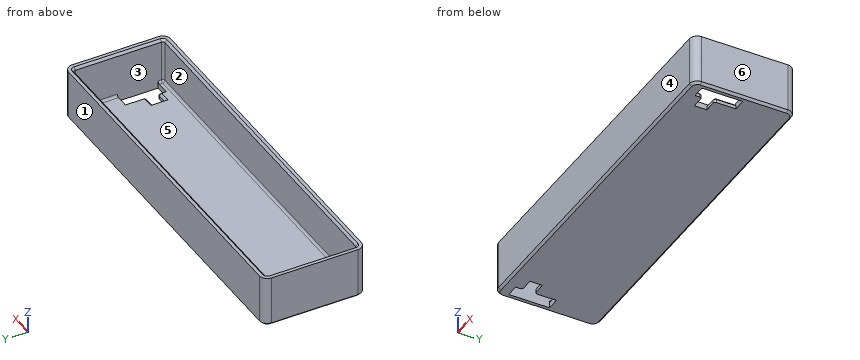
from build123d import *

# Parameters (mm, degrees)
SKETCH_W        = 154
SKETCH_H        = 40
PAD_DEPTH       = 2.5
SKETCH001_W     = 154
SKETCH001_H     = 22.5
PAD001_DEPTH    = 2.5
SKETCH002_W     = 154
SKETCH002_H     = 22.5
PAD002_DEPTH    = 2.5
SKETCH003_W     = 45
SKETCH003_H     = 22.5
PAD003_DEPTH    = 2.5
SKETCH004_W     = 45
SKETCH004_H     = 22.5
PAD004_DEPTH    = 2.5
SKETCH005_W     = 5.5
SKETCH005_H     = 18
POCKET_DEPTH    = 5
SKETCH006_W     = 6
SKETCH006_H     = 5.5
POCKET001_DEPTH = 5
FILLET_R        = 1
CHAMFER_SIZE    = 1
FILLET001_R     = 1
CHAMFER001_SIZE = 1
FILLET002_R     = 1
FILLET003_R     = 3.5
CHAMFER002_SIZE = 1
CHAMFER003_SIZE = 1


with BuildPart() as part:
    # Sketch → Pad (new body)
    with BuildSketch(Plane.XY):
        Rectangle(SKETCH_W, SKETCH_H)
    extrude(amount=PAD_DEPTH)

    # Sketch001 (on Face2 of Pad) → Pad001 (join)
    with BuildSketch(Plane.XZ.offset(20)):
        with Locations((0, 11.25)):
            Rectangle(SKETCH001_W, SKETCH001_H)
    extrude(amount=PAD001_DEPTH)

    # Sketch002 (on Face1 of Pad001) → Pad002 (join)
    with BuildSketch(Plane(origin=(0, 20, 0), x_dir=(-1, 0, 0), z_dir=(0, 1, 0))):
        with Locations((0, 11.25)):
            Rectangle(SKETCH002_W, SKETCH002_H)
    extrude(amount=PAD002_DEPTH)

    # Sketch003 (on Face9 of Pad002) → Pad003 (join)
    with BuildSketch(Plane.YZ.offset(77)):
        with Locations((0, 11.25)):
            Rectangle(SKETCH003_W, SKETCH003_H)
    extrude(amount=PAD003_DEPTH)

    # Sketch004 (on Face4 of Pad003) → Pad004 (join)
    with BuildSketch(Plane(origin=(-77, 0, 0), x_dir=(0, -1, 0), z_dir=(-1, 0, 0))):
        with Locations((0, 11.25)):
            Rectangle(SKETCH004_W, SKETCH004_H)
    extrude(amount=PAD004_DEPTH)

    # Sketch005 (on Face10 of Pad004) → Pocket (cut)
    with BuildSketch(Plane.XY.offset(2.5)):
        with Locations((-74.25, -8.5)):
            Rectangle(SKETCH005_W, SKETCH005_H)
        with Locations((74.25, -8.5)):
            Rectangle(SKETCH005_W, SKETCH005_H)
    extrude(amount=-POCKET_DEPTH, mode=Mode.SUBTRACT)

    # Sketch006 (on Face15 of Pocket) → Pocket001 (cut)
    with BuildSketch(Plane.XY.offset(2.5)):
        with Locations((-68.5, -11.75)):
            Rectangle(SKETCH006_W, SKETCH006_H)
        with Locations((68.5, -11.75)):
            Rectangle(SKETCH006_W, SKETCH006_H)
    extrude(amount=-POCKET001_DEPTH, mode=Mode.SUBTRACT)

    # Fillet
    fillet_edges = [part.edges().sort_by_distance(p)[0] for p in [
        (71.5, -9, 1.25),
        (71.5, -14.5, 1.25),
    ]]
    fillet(fillet_edges, radius=FILLET_R)

    # Chamfer
    chamfer_edges = [part.edges().sort_by_distance(p)[0] for p in [
        (68, -9, 2.5),
        (68, -14.5, 2.5),
    ]]
    chamfer(chamfer_edges, length=CHAMFER_SIZE)

    # Fillet001
    fillet001_edges = [part.edges().sort_by_distance(p)[0] for p in [
        (-71.5, -14.5, 1.25),
        (-71.5, -9, 1.25),
    ]]
    fillet(fillet001_edges, radius=FILLET001_R)

    # Chamfer001
    chamfer001_edges = [part.edges().sort_by_distance(p)[0] for p in [
        (-68, -14.5, 2.5),
        (-68, -9, 2.5),
    ]]
    chamfer(chamfer001_edges, length=CHAMFER001_SIZE)

    # Fillet002
    fillet002_edges = [part.edges().sort_by_distance(p)[0] for p in [
        (77, 20, 12.5),
        (77, 10.25, 2.5),
        (0, 20, 2.5),
        (77, -18.75, 2.5),
        (77, -20, 12.5),
        (0, -20, 2.5),
        (-77, 20, 12.5),
        (-77, 10.25, 2.5),
        (-77, -18.75, 2.5),
        (-77, -20, 12.5),
    ]]
    fillet(fillet002_edges, radius=FILLET002_R)

    # Fillet003
    fillet003_edges = [part.edges().sort_by_distance(p)[0] for p in [
        (-79.5, 22.5, 11.25),
        (-79.5, -22.5, 11.25),
        (79.5, -22.5, 11.25),
        (79.5, 22.5, 11.25),
    ]]
    fillet(fillet003_edges, radius=FILLET003_R)

    # Chamfer002
    chamfer002_edges = [part.edges().sort_by_distance(p)[0] for p in [
        (0, 22.5, 0),
    ]]
    chamfer(chamfer002_edges, length=CHAMFER002_SIZE)

    # Chamfer003
    chamfer003_edges = [part.edges().sort_by_distance(p)[0] for p in [
        (0, 20, 22.5),
    ]]
    chamfer(chamfer003_edges, length=CHAMFER003_SIZE)


solid = part.part
Could you check a few things on this model? Use its own coordinates, in mm. Face numbers are marked on the shaded views. A direction names the side the tool comes from. Give positions to 0.01 mm unless a question says otherwise; leave off trailing zeros. Order: outer loops, then holes, each group sorted by start corner. A loop starts at its lowest first (then second) coordinate and runs counter-clockwise, first axis right, second up. Notation, with made-up numbers: (53, 80.5) - (75, 80.5) arc R19 ccw to (75, 111.5) - close; hole circle Ø8 at (59, 23.5). An arc over 180 degrees is marked (long way). Return JSON: item names as keys, results as strings. Group by question number.
Q1. Suppose I cut it at D-D, the plane y = -11. Please give me the cut outline in (x, z).
Q2. Please list where these lines run through material, in increasing order: line 1 along X through (y, z) = (-11, 6.5); line 2 along Y through (x, z) = (-31, 19.75); line 3 along Z through (x, y) = (18, 18). Write a range as [from, to].
Q3. Suppose I cut it at C-C, the plane x = -40.5. Please give me the cut outline in (y, z).
Q4. Suppose I cut it at A-A, the plane z = 14. Please give me the cut outline in (x, y).
Q5. Will these pins go through, and if not, where does the flat tip stop? pin 1 Ø1.7 at (x, z) = (68, 0.5) entering from -Y; pin 2 Ø11.5 at (x, y) = (22, -8.5) entering from +Z.
Q6. Which directions (+Z, -Z, +X, -X, +Y, -Y) give clear straight access to the entire face, cutting with the end or side of a thin tool? Please do the marked faces 5 and 6.
Q7. Thinking about a two-plate mould opening in Y: for the marked faces 1, 2, 3 and 4, which applies, pulls with the +Y half, pulls with the -Y half, needs draft (parallel to the pull), parting line crosses it, or undercut?
Q8. Suppose I cut it at B-B, the plane y = -4.5. Please give me the cut outline in (x, z), and give its area (3 significant figures).
Resolved:
{
 "1": {"outline": "(-79.5, 1) - (-78.5, 0) - (-77, 0) - (-77, 21.5) - (-78, 22.5) - (-79.5, 22.5) - close; (-65.5, 0) - (65.5, 0) - (65.5, 2.5) - (-65.5, 2.5) - close; (77, 0) - (78.5, 0) - (79.5, 1) - (79.5, 22.5) - (78, 22.5) - (77, 21.5) - close"},
 "2": {"line 1": "x = [-79.5, -77], [77, 79.5]", "line 2": "y = [-22.5, -20], [20, 22.5]", "line 3": "z = [0, 2.5]"},
 "3": {"outline": "(-22.5, 1) - (-21.5, 0) - (21.5, 0) - (22.5, 1) - (22.5, 22.5) - (21, 22.5) - (20, 21.5) - (20, 3.5) arc R1 cw to (19, 2.5) - (-19, 2.5) arc R1 cw to (-20, 3.5) - (-20, 21.5) - (-21, 22.5) - (-22.5, 22.5) - close"},
 "4": {"outline": "(-79.5, -19) arc R3.5 ccw to (-76, -22.5) - (76, -22.5) arc R3.5 ccw to (79.5, -19) - (79.5, 19) arc R3.5 ccw to (76, 22.5) - (-76, 22.5) arc R3.5 ccw to (-79.5, 19) - close; hole (-77, -19) arc R1 ccw to (-76, -20) - (76, -20) arc R1 ccw to (77, -19) - (77, 19) arc R1 ccw to (76, 20) - (-76, 20) arc R1 ccw to (-77, 19) - close"},
 "5": {"pin 1": "stops at y = -22.5", "pin 2": "stops at z = 2.5"},
 "6": {"face 5": "+Z", "face 6": "+Z, -Z, +X, +Y, -Y"},
 "7": {"face 1": "pulls with the +Y half", "face 2": "undercut", "face 3": "undercut", "face 4": "pulls with the -Y half"},
 "8": {"outline": "(-79.5, 1) - (-78.5, 0) - (-77, 0) - (-77, 21.5) - (-78, 22.5) - (-79.5, 22.5) - close; (-71.5, 0) - (71.5, 0) - (71.5, 1.5) - (70.5, 2.5) - (-70.5, 2.5) - (-71.5, 1.5) - close; (77, 0) - (78.5, 0) - (79.5, 1) - (79.5, 22.5) - (78, 22.5) - (77, 21.5) - close", "area": "467 mm2"}
}
